Autodesk Inventor part; units mm, degrees
ref_plane "Work Plane1" through (0, 0, 0) normal (0, 0, -1) x (1, 0, 0)
ref_plane "YZ Plane" through (0, 0, 0) normal (1, 0, 0) x (0, 1, 0)
ref_plane "XZ Plane" through (0, 0, 0) normal (0, 1, 0) x (-1, 0, 0)
sketch "Sketch1" plane through (0, 0, 0) normal (0, 0, 1) x (1, 0, 0)
  line L0 (0, 0) -> (25.4, 0)
  line L1 (25.4, 0) -> (25.4, -25.4)
  line L2 (25.4, -25.4) -> (0, -25.4)
  line L3 (0, -25.4) -> (0, 0)
  dimension "d0" = 25.4
  dimension "d1" = 25.4
ref_plane "Work Plane1" through (0, 0, 0) normal (0, 0, -1) x (1, 0, 0)
sketch "Sketch2" plane through (0, 0, 0) normal (0, 0, -1) x (1, 0, 0)
  line L0 (1.524, 1.524) -> (23.876, 1.524)
  line L1 (23.876, 1.524) -> (23.876, 23.876)
  line L2 (23.876, 23.876) -> (1.524, 23.876)
  line L3 (1.524, 23.876) -> (1.524, 1.524)
  line L4 (0, 25.4) -> (0, 0)
  line L5 (0, 0) -> (25.4, 0)
  line L6 (25.4, 25.4) -> (0, 25.4)
  line L7 (25.4, 0) -> (25.4, 25.4)
  dimension "margin" = 1.524
  dimension "d3" = 1.524
  dimension "d4" = 1.524
  dimension "d5" = 1.524
extrude "Extrusion1" add sketch "Sketch2" along normal blind 127
equation "\"d3\" = margin"
equation "\"d4\" = margin"
equation "\"d5\" = margin"
properties part number "latch mount point"
Source: CAD feature listing. Evaluate the final solid. Frame: model axes, mm. A direction names the side the tool comes from. Give positions to 0.01 mm unless a question says otherwise; leave off trailing zeros. Order: outer loops, then holes, each group sorted by start corner. A loop starts at its lowest first (then second) coordinate and runs counter-clockwise, first axis right, second up. Notation, with made-up numbers: (6.5, 77.25) -> (35.5, 77.25) arc R25 ccw to (35.5, 96.25) -> close; hole circle Ø5 at (-26, 20.5). An arc over 180 degrees is marked (long way). Use a Markdown table: item, result.
1) Section query C-C, the plane x = 4. Return the cut outline in (y, z).
Answer list:
| item | result |
|---|---|
| outline | (-25.4, -127) -> (-23.88, -127) -> (-23.88, 0) -> (-25.4, 0) -> close; (-1.52, -127) -> (0, -127) -> (0, 0) -> (-1.52, 0) -> close |
2) Mould query, pull axis X, two halves, no side actions, for faces 1 (the flat face through (0, -13, -63)), 2 (the flat face through (1, -13, -127)), 3 (the flat face through (25.4, -13, -63)), 4 (the flat face through (1.524, -13, -63)). Classes: +X half, -X half, draft (parallel to the pull), parting line (faces both ways), or undercut.
Answer list:
| item | result |
|---|---|
| face 1 | -X half |
| face 2 | draft |
| face 3 | +X half |
| face 4 | undercut |
3) Reachability of faces 5 (the flat face through (23.876, -13, -63)), 6 (the flat face through (13, -25.4, -63)) from +Z, -Z, +X, -X, +Y, -Y: full face, straight path, thin tool, end or side. Return the list, or none.
Answer list:
| item | result |
|---|---|
| face 5 | +Z, -Z |
| face 6 | +Z, -Z, +X, -X, -Y |
4) Contact query for a flat-ended pin moving along its axis: P1, Ø1.5, axis at x = 21.5, y = -22.5, coming from the -Z side. Output: stop coordinate, or through.
Answer list:
| item | result |
|---|---|
| P1 | through |
5) Section query B-B, the plane z = -77.5. Return the cut outline in (x, y), then the cut area to 3 significant figures.
Answer list:
| item | result |
|---|---|
| outline | (0, -25.4) -> (25.4, -25.4) -> (25.4, 0) -> (0, 0) -> close; hole (1.52, -23.88) -> (23.88, -23.88) -> (23.88, -1.52) -> (1.52, -1.52) -> close |
| area | 146 mm² |
6) Ray query, line 1 along X through (y, z) = (-22.5, -13.5); line 2 along Y through (x, z) = (20, -23.5). Return the intervals inside material, ascending. Write a range as [from, to].
Answer list:
| item | result |
|---|---|
| line 1 | [0, 1.52], [23.88, 25.4] |
| line 2 | [-25.4, -23.88], [-1.52, 0] |
7) Section query A-A, the plane y = -13.75. Return the cut outline in (x, z).
Answer list:
| item | result |
|---|---|
| outline | (0, -127) -> (1.52, -127) -> (1.52, 0) -> (0, 0) -> close; (23.88, -127) -> (25.4, -127) -> (25.4, 0) -> (23.88, 0) -> close |
